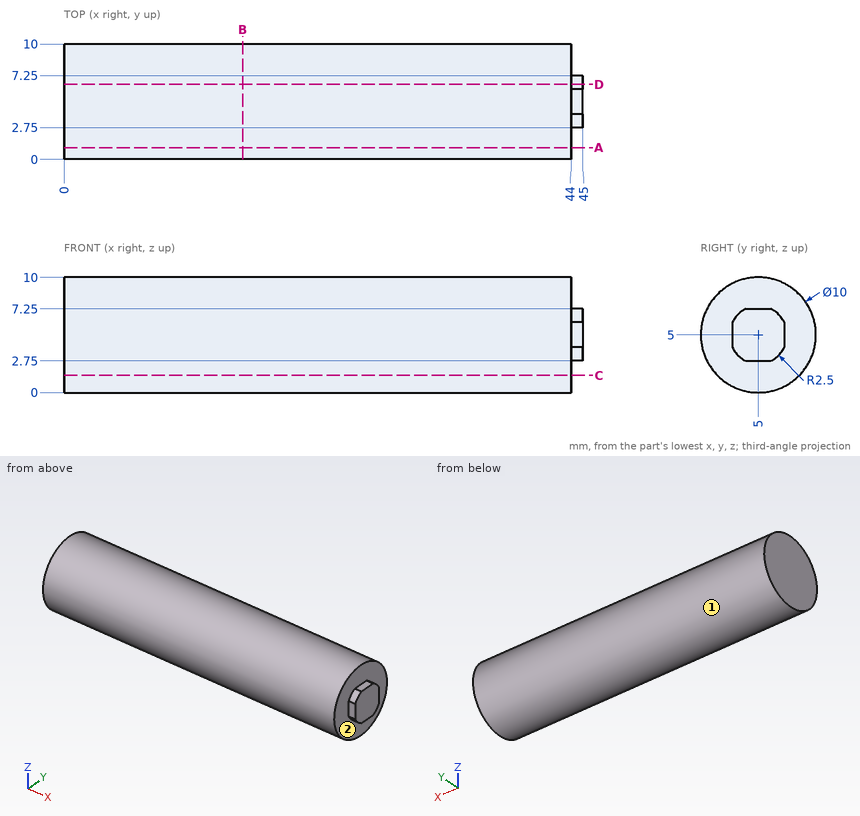
Drawing for the job (mm, zero at the part's lowest x, y, z). A direction names the side the tool comes from. Round coordinates to 2 decimals unless told otherwise and drop trailing zeros. Loops run counter-clockwise (first coordinate to the right, second up) from the corner with the lowest first, then second, coordinate; pieces in that order, holes last. Notation, with made-up numbers: (-8.5, 71.25) -> (37.5, 71.25) arc R19 cw to (37.5, 102.25) -> close; hole circle Ø8 at (-20.75, -32.5). An arc over 180 degrees is marked (long way). Use one line per item in the form item = value. Start each with the question number.
Item 1: Tool access for the marked faces 1 and 2: list every direction of +Z, -Z, +X, -X, +Y, -Y with a clear straight run to the whole face (end or side of a thin tool).
Item 2: Band-saw the part on A-A (y = 1). List the corners of the cut face in (x, z).
Item 3: Band-saw the part on B-B (x = 15.5). List the corners of the cut face in (y, z), plus the area to 3 significant figures.
Item 4: Drill centre lines: line 1 along X through (y, z) = (2.25, 8.25); line 2 along Y through (x, z) = (42, 4.75). Where is each one in solid material? Low to high.
Item 5: Drop flat-ended pins along their axis: pin 1 Ø0.8 at (x, y) = (44.5, 4.5) entering from -Z; pin 2 Ø0.8 at (x, z) = (44.5, 5) entering from +Y; pin 3 Ø3 at (x, y) = (28, 1) entering from -Z. Give the stop position or say it passes through.
Item 6: Band-saw the part on D-D (y = 6.5). List the corners of the cut face in (x, z), plus the area to 3 significant figures.
Item 7: Band-saw the part on C-C (z = 1.5). List the corners of the cut face in (x, y).
Data:
q1.face_1 = +X, -X
q1.face_2 = +X
q2.outline = (0, 2) -> (44, 2) -> (44, 8) -> (0, 8) -> close
q3.outline = circle Ø10 at (5, 5)
q3.area = 78.5 mm^2
q4.line_1 = 0 to 44
q4.line_2 = 0.01 to 9.99
q5.pin_1 = 2.75
q5.pin_2 = 7.25
q5.pin_3 = 0.67
q6.outline = (0, 0.23) -> (44, 0.23) -> (44, 3) -> (45, 3) -> (45, 7) -> (44, 7) -> (44, 9.77) -> (0, 9.77) -> close
q6.area = 424 mm^2
q7.outline = (0, 1.43) -> (44, 1.43) -> (44, 8.57) -> (0, 8.57) -> close
